```python
from build123d import *

# Parameters (mm, degrees)
F0_R      = 35
F1_DEPTH  = 25
F2_W      = 70
F2_H      = 10
F3_DEPTH  = 15
F5_W      = 8
F5_H      = 12
F6_DEPTH  = 25
F7_R      = 2.5
F8_DEPTH  = 50
F10_DEPTH = 2
F11_SIZE  = 1


with BuildPart() as f1:
    # F0 (on Top) → F1 (new body)
    with BuildSketch(Plane.XY):
        Circle(F0_R)
    extrude(amount=F1_DEPTH)

    # F2 (on face) → F3 (cut)
    with BuildSketch(Plane.XY.offset(25)):
        Rectangle(F2_W, F2_H)
    extrude(amount=-F3_DEPTH, mode=Mode.SUBTRACT)

    # F5 (on offset) → F6 (cut)
    with BuildSketch(Plane.XZ.offset(15)):
        Polygon((58, 13), (58, 33), (23, 33), (23, 21), (23, 13), align=None)
        with Locations((19, 27)):
            Rectangle(F5_W, F5_H)
        with BuildLine():
            Line((23, 13), (23, 21))
            Line((23, 21), (15, 21))
            ThreePointArc((15, 21), (17.3431457505, 15.3431457505), (23, 13))
        make_face()
    extrude(amount=F6_DEPTH, mode=Mode.SUBTRACT)

    # F7 (on face) → F8 (cut)
    with BuildSketch(Plane.XZ.offset(15)):
        with Locations((21.6227766017, 20)):
            Circle(F7_R)
    extrude(amount=-F8_DEPTH, mode=Mode.SUBTRACT)

    # F9 (on face) → F10 (cut)
    with BuildSketch(Plane(origin=(0, 0, 0), x_dir=(1, 0, 0), z_dir=(0, 0, -1))):
        with BuildLine():
            ThreePointArc((29.7321374946, -4), (29.9329594664, -2.0044793789), (30, 0))
            ThreePointArc((30, 0), (29.9329594664, 2.0044793789), (29.7321374946, 4))
            Line((29.7321374946, 4), (29.7321374946, -4))
        make_face()
        with BuildLine():
            ThreePointArc((29.7321374946, 4), (29.9329594664, 2.0044793789), (30, 0))
            ThreePointArc((30, 0), (29.9329594664, -2.0044793789), (29.7321374946, -4))
            Line((29.7321374946, -4), (35.7321374946, -4))
            Line((35.7321374946, -4), (35.7321374946, 4))
            Line((35.7321374946, 4), (29.7321374946, 4))
        make_face()
        with BuildLine():
            Line((29.7321374946, -4), (29.7321374946, 4))
            ThreePointArc((29.7321374946, 4), (21.2132034356, 21.2132034356), (4, 29.7321374946))
            Line((4, 29.7321374946), (-4, 29.7321374946))
            ThreePointArc((-4, 29.7321374946), (-21.2132034356, 21.2132034356), (-29.7321374946, 4))
            Line((-29.7321374946, 4), (-29.7321374946, -4))
            ThreePointArc((-29.7321374946, -4), (-21.2132034356, -21.2132034356), (-4, -29.7321374946))
            Line((-4, -29.7321374946), (4, -29.7321374946))
            ThreePointArc((4, -29.7321374946), (21.2132034356, -21.2132034356), (29.7321374946, -4))
        make_face()
        with BuildLine():
            Line((-4, 29.7321374946), (4, 29.7321374946))
            ThreePointArc((4, 29.7321374946), (0, 30), (-4, 29.7321374946))
        make_face()
        with BuildLine():
            ThreePointArc((-4, 29.7321374946), (0, 30), (4, 29.7321374946))
            Line((4, 29.7321374946), (4, 35.7321374946))
            Line((4, 35.7321374946), (-4, 35.7321374946))
            Line((-4, 35.7321374946), (-4, 29.7321374946))
        make_face()
        with BuildLine():
            Line((4, -35.7321374946), (4, -29.7321374946))
            ThreePointArc((4, -29.7321374946), (0, -30), (-4, -29.7321374946))
            Line((-4, -29.7321374946), (-4, -35.7321374946))
            Line((-4, -35.7321374946), (4, -35.7321374946))
        make_face()
        with BuildLine():
            ThreePointArc((-4, -29.7321374946), (0, -30), (4, -29.7321374946))
            Line((4, -29.7321374946), (-4, -29.7321374946))
        make_face()
        with BuildLine():
            Line((-29.7321374946, -4), (-29.7321374946, 4))
            ThreePointArc((-29.7321374946, 4), (-30, 0), (-29.7321374946, -4))
        make_face()
        with BuildLine():
            ThreePointArc((-29.7321374946, -4), (-30, 0), (-29.7321374946, 4))
            Line((-29.7321374946, 4), (-35.7321374946, 4))
            Line((-35.7321374946, 4), (-35.7321374946, -4))
            Line((-35.7321374946, -4), (-29.7321374946, -4))
        make_face()
    extrude(amount=-F10_DEPTH, mode=Mode.SUBTRACT)

    # F11
    f11_edges = [f1.edges().sort_by_distance(p)[0] for p in [
        (21.213203, -21.213203, 0),
        (-21.213203, -21.213203, 0),
        (21.213203, 21.213203, 0),
        (-21.213203, 21.213203, 0),
        (-32.251407, -4, 0),
        (-32.251407, 4, 0),
        (-4, -32.251407, 0),
        (4, -32.251407, 0),
        (32.251407, -4, 0),
        (32.251407, 4, 0),
        (4, 32.251407, 0),
        (-4, 32.251407, 0),
    ]]
    chamfer(f11_edges, length=F11_SIZE)


solid = f1.part
```
The model under review builds one solid part; all positions refer to its coordinate system, in mm. A direction names the side the tool comes from. Round coordinates to 2 decimals unless told otherwise and drop trailing zeros. Order: outer loops, then holes, each group sorted by start corner. A loop starts at its lowest first (then second) coordinate and runs counter-clockwise, first axis right, second up. Notation, with made-up numbers: (51, -9.5) -> (83, -9.5) arc R26 cw to (83, 20.5) -> close; hole circle Ø7 at (49.25, 40.5). An arc over 180 degrees is marked (long way). Use a Markdown table: item, result.
Q1. We need section B-B on z = 20. Write out the cut boundary in (x, y), then the cut area to 3 significant figures.
Values:
| item | result |
|---|---|
| outline | (-34.64, -5) arc R35 ccw to (15.06, -31.59) -> (15.06, -15) -> (19.12, -15) -> (19.12, -5) -> close; (-34.64, 5) -> (19.12, 5) -> (19.12, 29.31) arc R35 ccw to start; (24.12, -15) -> (31.62, -15) arc R35 ccw to (34.64, -5) -> (24.12, -5) -> close; (24.12, 5) -> (34.64, 5) arc R35 ccw to (24.12, 25.36) -> close |
| area | 2,820 mm^2 |
Q2. Mouldability with a two-part tool opening along X and no side actions: class faces 6 (the conical face through (21.13, 21.52, 0.84)), 7 (the cylindrical face through (21.019, 21.406, 1.493)), 8 (the flat face through (23, 22, 0)), 9 (the cylindrical face through (17.281, -23.195, 15.406)) as +X half, -X half, draft (parallel to the pull), parting line (faces both ways), or undercut.
Values:
| item | result |
|---|---|
| face 6 | undercut |
| face 7 | undercut |
| face 8 | draft |
| face 9 | +X half |
Q3. Clearance check with flat-ended pins moving along their axes: P1, Ø4, axis at x = -4, z = 3.5, coming from the -Y side; P2, Ø4.5, axis at x = 4.5, z = 17.5, coming from the +Y side; P3, Ø2, axis at x = -21, z = 3.5, coming from the +Y side. State where each tip first meets the part, or that it passes through.
Values:
| item | result |
|---|---|
| P1 | stops at y = -34.94 |
| P2 | stops at y = 34.93 |
| P3 | stops at y = 28.72 |
Q4. Tool access review of faces 1 (the flat face through (0, 0, 10)), 2 (the cylindrical face through (-21.406, 21.019, 1.493)), 3 (the flat face through (-22, -23, 0)), 4 (the flat face through (25, -15, 19)), 5 (the flat face through (0, 17, 25)): name each direction out of +Z, -Z, +X, -X, +Y, -Y from which nothing blocks a thin tool from reaching the whole face with its end or side.
Values:
| item | result |
|---|---|
| face 1 | +Z, +X, -X |
| face 2 | -Z |
| face 3 | -Z, +X, -X, +Y, -Y |
| face 4 | +Z, +X, -Y |
| face 5 | +Z, +X, -X, +Y, -Y |
Q5. We need section A-A on x = 0. Write out the cut boundary in (y, z), then the cut area to 3 significant figures.
Values:
| item | result |
|---|---|
| outline | (-35, 2) -> (35, 2) -> (35, 25) -> (5, 25) -> (5, 10) -> (-5, 10) -> (-5, 25) -> (-35, 25) -> close |
| area | 1,460 mm^2 |
Q6. For line 1 (Y direction, x = 17, z = 17.25); line 2 (Y direction, x = 1, z = 18.75); line 3 (Z direction, x = 19, y = -13), list the stretches that pass through material, from the lowest coordinate up.
Values:
| item | result |
|---|---|
| line 1 | y = -15 to -5, 5 to 30.59 |
| line 2 | y = -34.99 to -5, 5 to 34.99 |
| line 3 | z = 2 to 25 |
